from build123d import *

# Parameters (mm, degrees)
BOX181_W               = 0.8
BOX181_H               = 13
BOX181_DEPTH           = 0.8
BOX182_W               = 0.8
BOX182_H               = 13
BOX182_DEPTH           = 0.8
CUT094_PLACEMENT_ANGLE = 170


with BuildPart() as cubo181:
    # Box181 → Box181 (new body)
    with BuildSketch(Plane.XY):
        with Locations((0.4, 6.5)):
            Rectangle(BOX181_W, BOX181_H)
    extrude(amount=BOX181_DEPTH)


with BuildPart() as obj1:
    # Box182 → Box182 (new body)
    with BuildSketch(Plane(origin=(0.3, 0, 0.3), x_dir=(1, 0, 0), z_dir=(0, 0, 1))):
        with Locations((0.4, 6.5)):
            Rectangle(BOX182_W, BOX182_H)
    extrude(amount=BOX182_DEPTH)

    # Cut094: cut Cubo181
    add(cubo181.part, mode=Mode.SUBTRACT)


with BuildPart() as obj1_1:
    # Cut094 placement: moved
    add(obj1.part.moved(Location((-136.5, 188.9, -1.45))).rotate(Axis((-136.5, 188.9, -1.45), (0, 0, 1)), CUT094_PLACEMENT_ANGLE))


solid = obj1_1.part
Source: CAD feature listing. Evaluate the final solid. Frame: model axes, mm. A direction names the side the tool comes from. Give positions to 0.01 mm unless a question says otherwise; leave off trailing zeros. Write each loop counter-clockwise with the first axis right and the second up, starting at its lowest first coordinate (ties: lowest second). Pieces come first, ordered by that corner, then holes. Notation, with made-up numbers: M 29.25,38.5 L 56.25,38.5 A25 ccw 56.25,65.5 Z; hole C 54.5,77.25 d2. An arc over 180 degrees is marked long. Answer as a JSON object with one key per item and string values.
Q1. Cut plane C-C, the plane y = 183. Return the cut outline in (x, z).
Geometry check:
{"outline": "M -138.66,-1.15 L -138.35,-1.15 L -138.35,-0.65 L -137.84,-0.65 L -137.84,-0.35 L -138.66,-0.35 Z"}
Q2. Cut plane B-B, the plane z = -0.8. Return the cut outline in (x, y).
Geometry check:
{"outline": "M -139.84,176.29 L -139.55,176.24 L -137.29,189.04 L -137.58,189.09 Z"}
Q3. Contact query for a flat-ended pin moving along its axis: P1, Ø1.4, axis at x = -138.5, y = 182, coming from the -Z side. Output: stop coordinate, or through.
Geometry check:
{"P1": "stops at z = -1.15"}
Q4. Access query for faces 1 (the face through (-138, 183, -0.65)), 2 (the face through (-138.696, 182.779, -0.756)). Directions: +Z, -Z, +X, -X, +Y, -Y. A direction counts if a zero-diameter tool reaches every point of the face in a straight line with its end or side. Return the directions, or none.
Geometry check:
{"face 1": "-Z, +X, -Y", "face 2": "+Z, -Z, -X, +Y"}
Q5. Ray query, line 1 along Z through (x, y) = (-138.65, 179); line 2 along X through (y, z) = (186.5, -0.5); line 3 along X through (y, z) = (181.5, -0.8). Return the intervals inside material, ascending.
Geometry check:
{"line 1": "z = -0.65 to -0.35", "line 2": "x = -138.04 to -137.23", "line 3": "x = -138.92 to -138.62"}
Q6. Cut plane A-A, the plane x = -139.35. Return the cut outline in (y, z), then the cut area to 3 significant figures.
Geometry check:
{"outline": "M 176.2,-0.65 L 177.34,-0.65 L 177.34,-1.15 L 179.07,-1.15 L 179.07,-0.35 L 176.2,-0.35 Z", "area": "1.72 mm^2"}
